Source: CAD feature listing. Evaluate the final solid. Frame: model axes, mm. Face numbers are marked on the shaded views. A direction names the side the tool comes from. Coordinates: 2 decimals unless noted, no trailing zeros. Order: outer loops, then holes, each group sorted by start corner. A loop starts at its lowest first (then second) coordinate and runs counter-clockwise, first axis right, second up. Notation, with made-up numbers: (5.25, 76) -> (54.25, 76) arc R19 cw to (54.25, 107) -> close; hole circle Ø8 at (58.5, 56.5). An arc over 180 degrees is marked (long way). Write item = value, one per line. Start each with the question number.
Item 1: Section query D-D (z = -10.5). Output: boundary loops of the cut face in (x, y).
Item 2: Mould query, pull axis Z, two halves, no side actions, for the marked faces 6, 7 and 8. Classes: released by +Z, released by -Z, zero draft, split by the parting line, or undercut.
Item 3: Ray query, line 1 along X through (y, z) = (10, 15.5) (3 decimals); line 2 along Y through (x, z) = (9, 10); line 3 along Z through (x, y) = (12.5, 15). Return the intervals inside material, ascending. Write a range as [from, to].
Item 4: Section query B-B (y = 23). Output: boundary loops of the cut face in (x, z) (3 decimals).
Item 5: Contact query for flat-ended pins moving along their axis: pin 1 (6 mm diameter, centred on x = -16.5, z = 2, fed in from +Y); pin 2 (0.8 mm diameter, centred on x = 0, z = 14, fed in from -Y); pin 3 (2 mm diameter, centred on y = 15, z = -14, fed in from -X); pin 4 (0.7 mm diameter, centred on y = 18, z = -14.5, fed in from +X). Output: stop coordinate, or through.
Item 6: Section query A-A (x = 0). Output: boundary loops of the cut face in (y, z).
Item 7: Section query C-C (x = -10). Output: boundary loops of the cut face in (y, z).
Item 8: Set-up query: the marked faces 1, 2, 3, 4 and 5. Return all of +Z, -Z, +X, -X, +Y, -Y with unobstructed straight access to the full face (end or side cutting, diameter ignored); none if empty.
```python
from build123d import *

# Parameters (mm, degrees)
BOSS_EXTRUDE5_DEPTH = 32
CUT_EXTRUDE1_DEPTH  = 31
CUT_EXTRUDE2_DEPTH  = 45.879317341
CUT_EXTRUDE3_START  = -15
CUT_EXTRUDE3_DEPTH  = 2
FILLET1_R           = 4
FILLET2_R           = 2
CUT_EXTRUDE4_DEPTH  = 77.779196401
CUT_EXTRUDE5_DEPTH  = 55


with BuildPart() as part:
    # Sketch1 → Boss-Extrude5 (new body)
    with BuildSketch(Plane(origin=(0, 0, 0), x_dir=(1, 0, 0), z_dir=(0, 1, 0))):
        with BuildLine():
            Line((-0.399762594, -21.65), (18.175, -21.65))
            ThreePointArc((18.175, -21.65), (21.003427125, -20.478427125), (22.175, -17.65))
            Line((22.175, -17.65), (22.175, -8.65))
            Line((22.175, -8.65), (22.175, 6.65))
            ThreePointArc((22.175, 6.65), (19.538961031, 13.013961031), (13.175, 15.65))
            Line((13.175, 15.65), (-15.175, 15.65))
            ThreePointArc((-15.175, 15.65), (-21.538961031, 13.013961031), (-24.175, 6.65))
            Line((-24.175, 6.65), (-24.175, -8.65))
            Line((-24.175, -8.65), (-24.175, -17.65))
            ThreePointArc((-24.175, -17.65), (-23.003427125, -20.478427125), (-20.175, -21.65))
            Line((-20.175, -21.65), (-1.758134267, -21.65))
            Line((-1.758134267, -21.65), (-1.758134267, -19.65))
            Line((-1.758134267, -19.65), (-19.175, -19.65))
            ThreePointArc((-19.175, -19.65), (-21.296320344, -18.771320344), (-22.175, -16.65))
            Line((-22.175, -16.65), (-22.175, -14.65))
            Line((-22.175, -14.65), (20.175, -14.65))
            Line((20.175, -14.65), (20.175, -16.65))
            ThreePointArc((20.175, -16.65), (19.296320344, -18.771320344), (17.175, -19.65))
            Line((17.175, -19.65), (-0.399762594, -19.65))
            Line((-0.399762594, -19.65), (-0.399762594, -21.65))
        make_face()
    extrude(amount=BOSS_EXTRUDE5_DEPTH)

    # Sketch6 → Cut-Extrude1 (cut)
    with BuildSketch(Plane(origin=(0, 32, 0), x_dir=(1, 0, 0), z_dir=(0, 1, 0))):
        with BuildLine():
            Line((-14.175, 13.65), (12.175, 13.65))
            ThreePointArc((12.175, 13.65), (17.831854249, 11.306854249), (20.175, 5.65))
            Line((20.175, 5.65), (20.175, -5.65))
            ThreePointArc((20.175, -5.65), (17.831854249, -11.306854249), (12.175, -13.65))
            Line((12.175, -13.65), (-14.175, -13.65))
            ThreePointArc((-14.175, -13.65), (-19.831854249, -11.306854249), (-22.175, -5.65))
            Line((-22.175, -5.65), (-22.175, 5.65))
            ThreePointArc((-22.175, 5.65), (-19.831854249, 11.306854249), (-14.175, 13.65))
        make_face()
    extrude(amount=-CUT_EXTRUDE1_DEPTH, mode=Mode.SUBTRACT)

    # Sketch9 → Cut-Extrude2 (cut, through all)
    with BuildSketch(Plane(origin=(0, 1, 0), x_dir=(1, 0, 0), z_dir=(0, 1, 0))):
        with BuildLine():
            Line((-12.175, 8.65), (10.175, 8.65))
            ThreePointArc((10.175, 8.65), (13.710533906, 7.185533906), (15.175, 3.65))
            Line((15.175, 3.65), (15.175, -3.65))
            ThreePointArc((15.175, -3.65), (13.710533906, -7.185533906), (10.175, -8.65))
            Line((10.175, -8.65), (-12.175, -8.65))
            ThreePointArc((-12.175, -8.65), (-15.710533906, -7.185533906), (-17.175, -3.65))
            Line((-17.175, -3.65), (-17.175, 3.65))
            ThreePointArc((-17.175, 3.65), (-15.710533906, 7.185533906), (-12.175, 8.65))
        make_face()
    extrude(amount=-CUT_EXTRUDE2_DEPTH, mode=Mode.SUBTRACT)

    # Sketch11 → Cut-Extrude3 (cut)
    with BuildSketch(Plane.XY.offset(34.65).offset(CUT_EXTRUDE3_START)):
        Polygon((-2.600625842, 32), (-11.175, 0), (0.600625842, 0), (9.175, 32), align=None)
    extrude(amount=CUT_EXTRUDE3_DEPTH, mode=Mode.SUBTRACT)

    # Fillet1
    fillet1_edges = [part.edges().sort_by_distance(p)[0] for p in [
        (0.600625842, 0, 20.65),
        (-2.600625842, 32, 20.65),
    ]]
    fillet(fillet1_edges, radius=FILLET1_R)

    # Fillet2
    fillet2_edges = [part.edges().sort_by_distance(p)[0] for p in [
        (9.175, 32, 20.65),
        (-11.175, 0, 20.65),
    ]]
    fillet(fillet2_edges, radius=FILLET2_R)

    # Sketch13 → Cut-Extrude4 (cut, through all)
    with BuildSketch(Plane.ZY.offset(44.175)):
        with BuildLine():
            Line((-9.65, 30.5), (10.65, 30.5))
            ThreePointArc((10.65, 30.5), (12.771320344, 29.621320344), (13.65, 27.5))
            Line((13.65, 27.5), (13.65, 5.5))
            ThreePointArc((13.65, 5.5), (12.771320344, 3.378679656), (10.65, 2.5))
            Line((10.65, 2.5), (-9.65, 2.5))
            ThreePointArc((-9.65, 2.5), (-11.771320344, 3.378679656), (-12.65, 5.5))
            Line((-12.65, 5.5), (-12.65, 27.5))
            ThreePointArc((-12.65, 27.5), (-11.771320344, 29.621320344), (-9.65, 30.5))
        make_face()
    extrude(amount=-CUT_EXTRUDE4_DEPTH, mode=Mode.SUBTRACT)

    # Sketch14 → Cut-Extrude5 (cut)
    with BuildSketch(Plane(origin=(0, 0, -35.65), x_dir=(-1, 0, 0), z_dir=(0, 0, -1))):
        with BuildLine():
            Line((-10.883203932, 27), (12.883203932, 27))
            ThreePointArc((12.883203932, 27), (16.418737838, 25.535533906), (17.883203932, 22))
            Line((17.883203932, 22), (17.883203932, 10))
            ThreePointArc((17.883203932, 10), (16.418737838, 6.464466094), (12.883203932, 5))
            Line((12.883203932, 5), (-10.883203932, 5))
            ThreePointArc((-10.883203932, 5), (-14.418737838, 6.464466094), (-15.883203932, 10))
            Line((-15.883203932, 10), (-15.883203932, 22))
            ThreePointArc((-15.883203932, 22), (-14.418737838, 25.535533906), (-10.883203932, 27))
        make_face()
    extrude(amount=-CUT_EXTRUDE5_DEPTH, mode=Mode.SUBTRACT)


solid = part.part
```
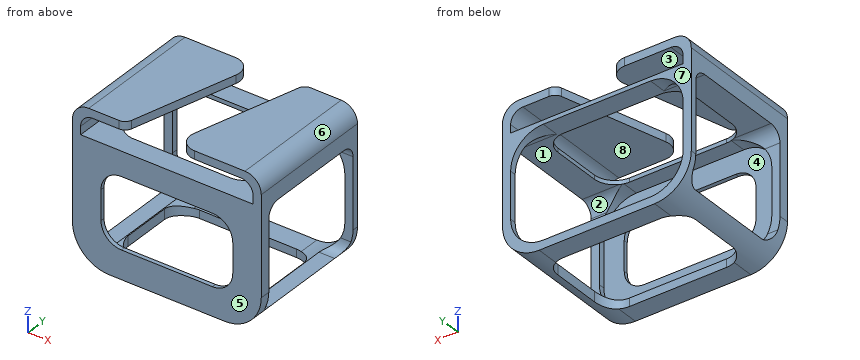
Computed:
q1.outline = (-23.31, 0) -> (21.31, 0) -> (21.31, 2.62) -> (18.54, 2.62) -> (18.54, 1) -> (-20.54, 1) -> (-20.54, 2.62) -> (-23.31, 2.62) -> close; (-23.31, 30.38) -> (-20.54, 30.38) -> (-20.54, 32) -> (-23.31, 32) -> close; (18.54, 30.38) -> (21.31, 30.38) -> (21.31, 32) -> (18.54, 32) -> close
q2.face_6 = released by +Z
q2.face_7 = zero draft
q2.face_8 = undercut
q3.line_1 = [-24.175, -22.175], [20.175, 22.175]
q3.line_2 = [0, 1]
q3.line_3 = [19.65, 21.65]
q4.outline = (-24.175, 13.65) -> (-17.782, 13.65) -> (-17.782, 14.65) -> (-22.175, 14.65) -> (-22.175, 16.65) arc R3 cw to (-19.175, 19.65) -> (-5.012, 19.65) -> (-5.012, 21.65) -> (-20.175, 21.65) arc R4 ccw to (-24.175, 17.65) -> close; (-21.883, -12.65) arc R9 ccw to (-17.782, -15.264) -> (-17.782, -12.791) arc R8 cw to (-18.048, -12.65) -> close; (6.763, 19.65) -> (17.175, 19.65) arc R3 cw to (20.175, 16.65) -> (20.175, 14.65) -> (15.782, 14.65) -> (15.782, 13.65) -> (22.175, 13.65) -> (22.175, 17.65) arc R4 ccw to (18.175, 21.65) -> (6.763, 21.65) -> close; (15.782, -15.264) arc R9 ccw to (19.883, -12.65) -> (16.048, -12.65) arc R8 cw to (15.782, -12.791) -> close
q5.pin_1 = 1
q5.pin_2 = 0
q5.pin_3 = -21.55
q5.pin_4 = 18.15
q6.outline = (0, -15.65) -> (5, -15.65) -> (5, -13.65) -> (1, -13.65) -> (1, -8.65) -> (0, -8.65) -> close; (0, 8.65) -> (1, 8.65) -> (1, 13.65) -> (5, 13.65) -> (5, 14.65) -> (0, 14.65) -> close; (27, -15.65) -> (32, -15.65) -> (32, -13.65) -> (27, -13.65) -> close; (27, 13.65) -> (32, 13.65) -> (32, 14.65) -> (27, 14.65) -> close
q7.outline = (0, -15.65) -> (5, -15.65) -> (5, -13.65) -> (1, -13.65) -> (1, -8.65) -> (0, -8.65) -> close; (0, 8.65) -> (1, 8.65) -> (1, 13.65) -> (5, 13.65) -> (5, 14.65) -> (0, 14.65) -> close; (4.39, 19.65) -> (32, 19.65) -> (32, 21.65) -> (4.39, 21.65) -> close; (27, -15.65) -> (32, -15.65) -> (32, -13.65) -> (27, -13.65) -> close; (27, 13.65) -> (32, 13.65) -> (32, 14.65) -> (27, 14.65) -> close
q8.face_1 = none
q8.face_2 = +X, -X
q8.face_3 = +Y, -Y
q8.face_4 = +Y
q8.face_5 = +Z, -Z, +X, -X, -Y
